Design review of the part built by this model. Coordinates are the model's own, in mm. A direction names the side the tool comes from. Give positions to 0.01 mm unless a question says otherwise; leave off trailing zeros. Order: outer loops, then holes, each group sorted by start corner. A loop starts at its lowest first (then second) coordinate and runs counter-clockwise, first axis right, second up. Notation, with made-up numbers: M 66.5,52 L 72.5,52 A8 ccw 72.5,65 Z; hole C 32.5,-19 d9. An arc over 180 degrees is marked long. Answer as a JSON object with one key per item and string values.
from build123d import *

# Parameters (mm, degrees)
F1_DEPTH  = 19
F2_DEPTH  = 5
F3_DEPTH  = 50
F5_DEPTH  = 45.001
F6_R      = 19
F6_R_2    = 8
F7_DEPTH  = 12
F8_DEPTH  = 13
F9_DEPTH  = 50
F10_R     = 8
F11_DEPTH = 10.001


with BuildPart() as f1:
    # F0 (on Right) → F1 (new body, symmetric)
    with BuildSketch(Plane.YZ):
        with BuildLine():
            Line((0, 0), (10, 0))
            Line((10, 0), (10, 30))
            ThreePointArc((10, 30), (11.464466, 33.535534), (15, 35))
            Line((15, 35), (88, 35))
            Line((88, 35), (88, 75))
            Line((88, 75), (78, 75))
            Line((78, 75), (78, 45))
            Line((78, 45), (15, 45))
            ThreePointArc((15, 45), (4.393398, 40.606602), (0, 30))
            Line((0, 30), (0, 0))
        make_face()
    extrude(amount=F1_DEPTH, both=True)

    # F0 (on Right) → F2 (join, symmetric)
    with BuildSketch(Plane.YZ):
        with BuildLine():
            Line((-10, 0), (0, 0))
            Line((0, 0), (0, 30))
            ThreePointArc((0, 30), (4.393398, 40.606602), (15, 45))
            Line((15, 45), (78, 45))
            Line((78, 45), (78, 75))
            ThreePointArc((78, 75), (69.316491, 60.635083), (53.505103, 55))
            Line((53.505103, 55), (15, 55))
            ThreePointArc((15, 55), (-2.67767, 47.67767), (-10, 30))
            Line((-10, 30), (-10, 0))
        make_face()
    extrude(amount=F2_DEPTH, both=True)

    # F0 (on Right) → F3 (join)
    with BuildSketch(Plane.YZ):
        with BuildLine():
            Line((0, 0), (10, 0))
            Line((10, 0), (10, 30))
            ThreePointArc((10, 30), (11.464466, 33.535534), (15, 35))
            Line((15, 35), (88, 35))
            Line((88, 35), (88, 75))
            Line((88, 75), (78, 75))
            Line((78, 75), (78, 45))
            Line((78, 45), (15, 45))
            ThreePointArc((15, 45), (4.393398, 40.606602), (0, 30))
            Line((0, 30), (0, 0))
        make_face()
    extrude(amount=-F3_DEPTH)

    # F4 (on face) → F5 (cut, through all)
    with BuildSketch(Plane.XY.offset(45)):
        with BuildLine():
            ThreePointArc((-19, 47), (-28.07969, 68.92031), (-50, 78))
            Line((-50, 78), (-50, 0))
            Line((-50, 0), (-19, 0))
            Line((-19, 0), (-19, 15))
            Line((-19, 15), (-19, 47))
        make_face()
    extrude(amount=-F5_DEPTH, mode=Mode.SUBTRACT)

    # F6 (on Front) → F7 (join)
    with BuildSketch(Plane.XZ):
        Circle(F6_R)
        Circle(F6_R_2, mode=Mode.SUBTRACT)
        Circle(F6_R_2)
    extrude(amount=F7_DEPTH)

    # F6 (on Front) → F8 (join)
    with BuildSketch(Plane.XZ):
        Circle(F6_R)
        Circle(F6_R_2, mode=Mode.SUBTRACT)
        Circle(F6_R_2)
    extrude(amount=-F8_DEPTH)

    # F6 (on Front) → F9 (cut, symmetric)
    with BuildSketch(Plane.XZ):
        Circle(F6_R_2)
    extrude(amount=F9_DEPTH, both=True, mode=Mode.SUBTRACT)

    # F10 (on face) → F11 (cut, through all)
    with BuildSketch(Plane.XZ.offset(-78)):
        with Locations((-28, 57)):
            Circle(F10_R)
    extrude(amount=-F11_DEPTH, mode=Mode.SUBTRACT)


solid = f1.part
(1) We need section A-A (x = 0). Write out the cut boundary in (y, z), plus the area to 3 significant figures.
Checked values:
{"outline": "M -12,-19 L 13,-19 L 13,-8 L -12,-8 Z; M -12,8 L 13,8 L 13,19 L 10,19 L 10,30 A5 cw 15,35 L 88,35 L 88,75 L 78,75 A25 cw 53.51,55 L 15,55 A25 ccw -10,30 L -10,19 L -12,19 Z", "area": "3,020 mm^2"}
(2) To check wall thickness, follow L1, parallel to Z at x = -28, y = 80; L2, parallel to Y at x = -40, z = 58.5; L3, parallel to Y at x = 7, z = 6.5. State the ranges of each line that lie inside material, in increasing order. Write a range as from..to.
Checked values:
{"L1": "z = 35..49, 65..75", "L2": "y = 78..88", "L3": "y = -12..13"}
(3) Insertion check: pin 1 (1.5 mm diameter, centred on x = -10.5, y = 23.5, fed in from +Z); pin 2 (3 mm diameter, centred on x = -10.5, z = 5.5, fed in from +Y); pin 3 (1.5 mm diameter, centred on x = -41, z = 32.5, fed in from +Y); pin 4 (5 mm diameter, centred on x = -2, z = 21.5, fed in from -Y). Each pin has a flat end and moves straight along its axis. Give the tip position at first contact, or say it passes through.
Checked values:
{"pin 1": "stops at z = 45", "pin 2": "stops at y = 13", "pin 3": "passes through", "pin 4": "stops at y = -10"}
(4) Draft analysis for pull direction X (two halves, no side actions). For faces 5 (the cylindrical face through (-1.73, 0.32, -7.81)), 6 (the flat face through (-5, 31, 47)), 7 (the flat face through (5, 31, 47)), 8 (the flat face through (8.2, 13, 0.3)), state which applies: +X half, -X half, draft (parallel to the pull), parting line (faces both ways), or undercut.
Checked values:
{"face 5": "undercut", "face 6": "-X half", "face 7": "+X half", "face 8": "draft"}
(5) We need section C-C (y = 42). Write out the cut boundary in (x, z).
Checked values:
{"outline": "M -19,35 L 19,35 L 19,45 L 5,45 L 5,55 L -5,55 L -5,45 L -19,45 Z"}
(6) We need section D-D (x = -28). Write out the cut boundary in (y, z), plus the area to 3 significant figures.
Checked values:
{"outline": "M 68.84,35 L 88,35 L 88,49 L 78,49 L 78,45 L 68.84,45 Z; M 78,65 L 88,65 L 88,75 L 78,75 Z", "area": "332 mm^2"}
(7) Tool access review of faces 1 (the flat face through (0, 10, 21)), 2 (the cylindrical face through (-11.9, 4.51, 40.72)), 3 (the flat face through (14, 0, 22)), 4 (the flat face through (-19, 18, 38)): name each direction out of +Z, -Z, +X, -X, +Y, -Y from which nothing blocks a thin tool from reaching the whole face with its end or side.
Checked values:
{"face 1": "+Y", "face 2": "+Z, -X, -Y", "face 3": "+Z, +X, -Y", "face 4": "+Z, -Z, -X, -Y"}
(8) We need section B-B (z = 4). Write out the cut boundary in (x, y), plus the area to 3 significant figures.
Checked values:
{"outline": "M -19,0 L -18.57,0 L -18.57,-12 L -6.93,-12 L -6.93,13 L -18.57,13 L -18.57,10 L -19,10 Z; M 6.93,-12 L 18.57,-12 L 18.57,0 L 19,0 L 19,10 L 18.57,10 L 18.57,13 L 6.93,13 Z", "area": "591 mm^2"}
